from build123d import *

# Parameters (mm, degrees)
F1_DEPTH = 65
F2_R     = 5.5
F3_DEPTH = 52.001
F4_W     = 46
F4_H     = 55
F5_DEPTH = 25
F7_DEPTH = 7.5
F8_R     = 7.5
F9_DEPTH = 3
F10_R    = 2.99999


# Not quite as in the source:
# - a fillet or chamfer is up to 0.001 mm smaller than in the source, because OpenCascade refuses the exact size
# - a feature names something its author has since deleted; it is built from what else it names


with BuildPart() as f1:
    # F0 (on Front) → F1 (new body, symmetric)
    with BuildSketch(Plane.XZ):
        Polygon((-23, 20), (23, 20), (23, -20), (26, -20), (26, 23), (-26, 23), (-26, -20), (-23, -20), align=None)
    extrude(amount=F1_DEPTH, both=True)

    # F2 (on face) → F3 (cut, through all)
    with BuildSketch(Plane.YZ.offset(26)):
        with Locations((50, 3)):
            Circle(F2_R)
        with BuildLine():
            Line((65, -20), (65, 10))
            ThreePointArc((65, 10), (56.2132034356, -11.2132034356), (35, -20))
            Line((35, -20), (65, -20))
        make_face()
        with BuildLine():
            ThreePointArc((63.1113759485, 20.4761893015), (64.5119654739, 18.161266652), (65, 15.5))
            Line((65, 15.5), (65, 23))
            Line((65, 23), (62.0370116692, 23))
            ThreePointArc((62.0370116692, 23), (62.6030536231, 21.7503800228), (63.1113759485, 20.4761893015))
        make_face()
        with BuildLine():
            ThreePointArc((57.5, 23), (60.5764086399, 22.3400080322), (63.1113759485, 20.4761893015))
            ThreePointArc((63.1113759485, 20.4761893015), (62.6030536231, 21.7503800228), (62.0370116692, 23))
            Line((62.0370116692, 23), (57.5, 23))
        make_face()
    extrude(amount=-F3_DEPTH, mode=Mode.SUBTRACT)

    # F4 (on face) → F5 (cut)
    with BuildSketch(Plane(origin=(0, 0, 20), x_dir=(1, 0, 0), z_dir=(0, 0, -1))):
        with Locations((0, -37.5)):
            Rectangle(F4_W, F4_H)
    extrude(amount=-F5_DEPTH, mode=Mode.SUBTRACT)

    # F6 (on Right) → F7 (join, symmetric)
    with BuildSketch(Plane.YZ):
        Polygon((-60, 48), (-60, 23), (-57, 23), (-57, 45), (-7.0310988843, 45), (1.7689011157, 23), (5, 23), (-5, 48), align=None)
    extrude(amount=F7_DEPTH, both=True)

    # F8 (on face) → F9 (join)
    with BuildSketch(Plane(origin=(-26, 0, 0), x_dir=(0, -1, 0), z_dir=(-1, 0, 0))):
        with BuildLine():
            Line((7.5, -20), (-27.5, -20))
            Line((-27.5, -20), (-27.5, -67))
            ThreePointArc((-27.5, -67), (-10, -49.5), (7.5, -67))
            Line((7.5, -67), (7.5, -20))
        make_face()
        with BuildLine():
            ThreePointArc((7.5, -67), (-10, -49.5), (-27.5, -67))
            ThreePointArc((-27.5, -67), (-10, -84.5), (7.5, -67))
        make_face()
        with Locations((-10, -67)):
            Circle(F8_R, mode=Mode.SUBTRACT)
    extrude(amount=-F9_DEPTH)

    # F10 (radius 3 in the source; OpenCascade refuses exactly that, so slightly less here)
    f10_edges = [f1.edges().sort_by_distance(p)[0] for p in [
        (24.5, -65, -20),
        (-24.5, -65, -20),
        (0, -60, 48),
        (0, -57, 45),
        (0, -7.031099, 45),
        (0, -5, 48),
        (0, -65, 23),
    ]]
    fillet(f10_edges, radius=F10_R)


solid = f1.part
Source: CAD feature listing. Evaluate the final solid. Frame: model axes, mm. A direction names the side the tool comes from. Round coordinates to 2 decimals unless told otherwise and drop trailing zeros. Loops run counter-clockwise (first coordinate to the right, second up) from the corner with the lowest first, then second, coordinate; pieces in that order, holes last. Notation, with made-up numbers: (-34, 20) -> (-22, 20) arc R18 cw to (-22, 36) -> close; hole circle Ø7 at (74, 69). An arc over 180 degrees is marked (long way). Answer as a JSON object with one key per item and string values. Group by question number.
Q1. Mould query, pull axis Y, two halves, no side actions, for faces 5 (the cylindrical face through (-24.48, -64.14, -19.1)), 6 (the flat face through (0, -30, 23)), 7 (the cylindrical face through (-24.479, 56.445, -10.979)), 8 (the flat face through (24, -14, -20)). Classes: pulls with the +Y half, pulls with the -Y half, needs draft (parallel to the pull), parting line crosses it, or undercut.
Q2. Access query for faces 1 (the flat face through (0, -60, 34)), 2 (the flat face through (0.11, -2.31, 33.2)), 3 (the flat face through (0, 10, 21)), 4 (the flat face through (-7.5, -30, 46)). Directions: +Z, -Z, +X, -X, +Y, -Y. A direction counts if a zero-diameter tool reaches every point of the face in a straight line with its end or side. Return the directions, or none.
Q3. Section query C-C (z = 3). Output: boundary loops of the cut face in (x, y), plus the area to 3 significant figures.
Q4. Contact query for flat-ended pins moving along their axis: P1, Ø23, axis at x = -8, y = -37.5, coming from the -Z side; P2, Ø10, axis at x = 7.5, y = 18, coming from the +Z side; P3, Ø8, axis at x = 20, y = 4.5, coming from the -Z side; P4, Ø12, axis at x = 1, z = 35, coming from the +Y side. Output: stop coordinate, or through.
Q5. Section query A-A (y = -22). Output: boundary loops of the cut face in (x, z).
Q6. Ray query, line 1 (X direction, y = 24, z = 3.5); line 2 (Z direction, x = -25, y = 10); line 3 (Z direction, x = -3.5, y = -14). Return the intervals inside material, ascending. Write a range as from..to.
Completed:
{
 "1": {"face 5": "pulls with the -Y half", "face 6": "undercut", "face 7": "pulls with the +Y half", "face 8": "needs draft"},
 "2": {"face 1": "+Z, +X, -X, -Y", "face 2": "+X, -X", "face 3": "+Z, -Z, +Y", "face 4": "+Z, -X, +Y, -Y"},
 "3": {"outline": "(-26, -65) -> (-23, -65) -> (-23, 44.5) -> (-26, 44.5) -> close; (-26, 55.5) -> (-23, 55.5) -> (-23, 64.17) -> (-26, 64.17) -> close; (23, -65) -> (26, -65) -> (26, 44.5) -> (23, 44.5) -> close; (23, 55.5) -> (26, 55.5) -> (26, 64.17) -> (23, 64.17) -> close", "area": "709 mm²"},
 "4": {"P1": "z = 20", "P2": "through", "P3": "z = -20", "P4": "y = 2.6"},
 "5": {"outline": "(-26, -20) -> (-23, -20) -> (-23, 20) -> (23, 20) -> (23, -20) -> (26, -20) -> (26, 23) -> (-26, 23) -> close; (-7.5, 45) -> (7.5, 45) -> (7.5, 48) -> (-7.5, 48) -> close"},
 "6": {"line 1": "-26..-23, 23..26", "line 2": "-84.5..-74.5, -59.5..23", "line 3": "20..23, 45..48"}
}
